Geometry check sheet. Reference: the model listing, model coordinates, mm. A direction names the side the tool comes from. Give positions to 0.01 mm unless a question says otherwise; leave off trailing zeros. Order: outer loops, then holes, each group sorted by start corner. A loop starts at its lowest first (then second) coordinate and runs counter-clockwise, first axis right, second up. Notation, with made-up numbers: M 20,46.5 L 45,46.5 A27 cw 45,84.5 Z; hole C 78,-18.75 d2. An arc over 180 degrees is marked long. Answer as CSV lines item,"result". Start each with the question number.
```python
from build123d import *

# Parameters (mm, degrees)
BOSS_EXTRUDE1_DEPTH     = 30
BOSS_EXTRUDE2_DEPTH     = 30
CUT_EXTRUDE1_DEPTH      = 30
CUT_EXTRUDE3_DEPTH      = 43
CUT_EXTRUDE3_DEPTH_BACK = 100
SKETCH4_W               = 74
SKETCH4_H               = 15


with BuildPart() as part:
    # Sketch1 → Boss-Extrude1 (new body)
    with BuildSketch(Plane(origin=(0, 0, 0), x_dir=(0, 1, 0), z_dir=(0, 0, 1))):
        Polygon((0, 0), (0, 300), (-25.477916399, 370), (-27.406279228, 372.298133329), (-25.108145898, 374.226496158), (-27.036508727, 376.524629488), (-24.738375398, 378.452992317), (-26.666738227, 380.751125646), (-24.368604898, 382.679488475), (-26.296967727, 384.977621805), (-23.998834397, 386.905984634), (-25.927197227, 389.204117963), (-23.629063897, 391.132480792), (-25.557426726, 393.430614121), (-23.259293397, 395.35897695), (-25.187656226, 397.65711028), (-22.889522897, 399.585473109), (-24.817885726, 401.883606438), (-22.519752396, 403.811969267), (-24.448115225, 406.110102597), (-22.149981896, 408.038465426), (-24.078344725, 410.336598755), (-21.780211396, 412.264961584), (-23.708574225, 414.563094914), (-21.410440895, 416.491457743), (-23.338803724, 418.789591072), (-21.040670395, 420.717953901), (-22.969033224, 423.01608723), (-20.670899895, 424.944450059), (-22.599262724, 427.242583389), (-20.301129394, 429.170946218), (-22.229492224, 431.469079547), (-19.931358894, 433.397442376), (-21.859721723, 435.695575706), (-19.561588394, 437.623938535), (-21.489951223, 439.922071864), (-19.191817894, 441.850434693), (-21.120180723, 444.148568022), (-18.822047393, 446.076930851), (-22.113893269, 450), (-61.371757942, 450), (-75.477916399, 370), (-50, 300), (-50, 0), (-25, -25), align=None)
    extrude(amount=BOSS_EXTRUDE1_DEPTH)

    # Sketch3 → Boss-Extrude2 (add)
    with BuildSketch(Plane.XY.offset(30)):
        with BuildLine():
            Line((3.535533906, -3.535533906), (14.100912029, -14.100912029))
            Line((14.100912029, -14.100912029), (15.179930074, -13.021893985))
            ThreePointArc((15.179930074, -13.021893985), (20.03858246, -15.472056871), (25.466397806, -15.857571781))
            ThreePointArc((25.466397806, -15.857571781), (25.980762114, -15), (26.466258908, -14.125761553))
            ThreePointArc((26.466258908, -14.125761553), (23.418485529, -9.61789303), (18.867256033, -6.635258079))
            ThreePointArc((18.867256033, -6.635258079), (19.318516526, -5.176380902), (19.657152064, -3.68732596))
            ThreePointArc((19.657152064, -3.68732596), (25.089949902, -3.37990307), (29.983333333, -0.999861101))
            ThreePointArc((29.983333333, -0.999861101), (30, 0), (29.983333333, 0.999861101))
            ThreePointArc((29.983333333, 0.999861101), (25.089949902, 3.37990307), (19.657152064, 3.68732596))
            ThreePointArc((19.657152064, 3.68732596), (19.318516526, 5.176380902), (18.867256033, 6.635258079))
            ThreePointArc((18.867256033, 6.635258079), (23.418485529, 9.61789303), (26.466258908, 14.125761553))
            ThreePointArc((26.466258908, 14.125761553), (25.980762114, 15), (25.466397806, 15.857571781))
            ThreePointArc((25.466397806, 15.857571781), (20.03858246, 15.472056871), (15.179930074, 13.021893985))
            ThreePointArc((15.179930074, 13.021893985), (14.142135624, 14.142135624), (13.021893985, 15.179930074))
            ThreePointArc((13.021893985, 15.179930074), (15.472056871, 20.03858246), (15.857571781, 25.466397806))
            ThreePointArc((15.857571781, 25.466397806), (15, 25.980762114), (14.125761553, 26.466258908))
            ThreePointArc((14.125761553, 26.466258908), (9.61789303, 23.418485529), (6.635258079, 18.867256033))
            ThreePointArc((6.635258079, 18.867256033), (5.176380902, 19.318516526), (3.68732596, 19.657152064))
            ThreePointArc((3.68732596, 19.657152064), (3.37990307, 25.089949902), (0.999861101, 29.983333333))
            ThreePointArc((0.999861101, 29.983333333), (0, 30), (-0.999861101, 29.983333333))
            ThreePointArc((-0.999861101, 29.983333333), (-3.37990307, 25.089949902), (-3.68732596, 19.657152064))
            ThreePointArc((-3.68732596, 19.657152064), (-5.176380902, 19.318516526), (-6.635258079, 18.867256033))
            ThreePointArc((-6.635258079, 18.867256033), (-9.61789303, 23.418485529), (-14.125761553, 26.466258908))
            ThreePointArc((-14.125761553, 26.466258908), (-15, 25.980762114), (-15.857571781, 25.466397806))
            ThreePointArc((-15.857571781, 25.466397806), (-15.472056871, 20.03858246), (-13.021893985, 15.179930074))
            ThreePointArc((-13.021893985, 15.179930074), (-14.142135624, 14.142135624), (-15.179930074, 13.021893985))
            ThreePointArc((-15.179930074, 13.021893985), (-20.03858246, 15.472056871), (-25.466397806, 15.857571781))
            ThreePointArc((-25.466397806, 15.857571781), (-25.980762114, 15), (-26.466258908, 14.125761553))
            ThreePointArc((-26.466258908, 14.125761553), (-23.418485529, 9.61789303), (-18.867256033, 6.635258079))
            ThreePointArc((-18.867256033, 6.635258079), (-19.318516526, 5.176380902), (-19.657152064, 3.68732596))
            ThreePointArc((-19.657152064, 3.68732596), (-25.089949902, 3.37990307), (-29.983333333, 0.999861101))
            ThreePointArc((-29.983333333, 0.999861101), (-29.995833044, 0.5), (-30, 0))
            Line((-30, 0), (-5, 0))
            ThreePointArc((-5, 0), (-1.913417162, -4.619397663), (3.535533906, -3.535533906))
        make_face()
    extrude(amount=-BOSS_EXTRUDE2_DEPTH)

    # Sketch3<6> → Cut-Extrude1 (cut)
    with BuildSketch(Plane.XY.offset(30)):
        with BuildLine():
            Line((0, 0), (3.535533906, -3.535533906))
            ThreePointArc((3.535533906, -3.535533906), (4.619397663, -1.913417162), (5, 0))
            ThreePointArc((5, 0), (0, 5), (-5, 0))
            Line((-5, 0), (0, 0))
        make_face()
        with BuildLine():
            ThreePointArc((-5, 0), (-1.913417162, -4.619397663), (3.535533906, -3.535533906))
            Line((3.535533906, -3.535533906), (0, 0))
            Line((0, 0), (-5, 0))
        make_face()
    extrude(amount=-CUT_EXTRUDE1_DEPTH, mode=Mode.SUBTRACT)

    # Sketch4 → Cut-Extrude3 (cut, two sides: drawn at the far end of the back side and taken through both)
    with BuildSketch(Plane.YZ.offset(-CUT_EXTRUDE3_DEPTH_BACK)):
        with Locations((12, 15)):
            Rectangle(SKETCH4_W, SKETCH4_H)
    extrude(amount=CUT_EXTRUDE3_DEPTH + CUT_EXTRUDE3_DEPTH_BACK, mode=Mode.SUBTRACT)


solid = part.part
```
Item 1: Draft check along X on faces 5 (the face through (23.5, -9.7, 26.3)), 6 (the face through (-3.36, 25.16, 3.8)), 7 (the face through (-19.96, 15.45, 26.3)), 8 (the face through (-450, -41, 15)). Enter one of: pulls with the +X half, pulls with the -X half, needs draft (parallel to the pull), parting line crosses it, or undercut.
Item 2: Depth check by flat-ended pin: pin 1 Ø12 at (x, z) = (-107, 14) entering from +Y; pin 2 Ø8 at (y, z) = (-38, 7) entering from +X; pin 3 Ø8 at (y, z) = (-33.5, 9) entering from +X; pin 4 Ø16.5 at (x, y) = (-14.5, 15) entering from -Z. Enter the tip coordinate at first touch or a pass-through.
Item 3: Section check A-A on x = -253. Record the boundary of the cut face in (y, z), then the cut area to 3 significant figures.
Item 4: Section check B-B on y = -68. Record the boundary of the cut face in (x, z).
Item 5: Access from +Z, -Z, +X, -X, +Y, -Y to the whole of each face (thin tool, end or side, straight path). Record for faces 1 (the face through (25.016, -3.399, 3.803)), 2 (the face through (-23.5, 9.7, 3.8)), 3 (the face through (23.4, 9.6, 3.8)), 4 (the face through (-38, -25, 15)).
Item 6: Scan lines: line 1 along X through (y, z) = (-37, 2.75); line 2 along Y through (x, z) = (-263, 5.25); line 3 along Y through (x, z) = (-33, 16.5). Record each from-to range of solid material in increasing order.
Numbers:
1,face 5,"pulls with the +X half"
1,face 6,"undercut"
1,face 7,"undercut"
1,face 8,"pulls with the -X half"
2,pin 1,"y = 0"
2,pin 2,"x = 16"
2,pin 3,"x = 20.5"
2,pin 4,"z = 0"
3,outline,"M -50,0 L 0,0 L 0,30 L -50,30 Z"
3,area,"1,500 mm2"
4,outline,"M -412.41,0 L -349.45,0 L -349.45,30 L -412.41,30 Z"
5,face 1,"+Z, -Z"
5,face 2,"+Z, -Z, -X"
5,face 3,"+Z, -Z, +X"
5,face 4,"+X, +Y"
6,line 1,"-450 to 13"
6,line 2,"-50 to 0"
6,line 3,"-50 to -25"
